Input: part model. Units: mm. Frame: model coordinates. A direction names the side the tool comes from. Round coordinates to 2 decimals unless told otherwise and drop trailing zeros. Loops run counter-clockwise (first coordinate to the right, second up) from the corner with the lowest first, then second, coordinate; pieces in that order, holes last.
(1) Cut plane C-C, the plane y = -10. Output: boundary loops of the cut face in (x, z), and give its area (3 significant figures).
(2) Cut plane D-D, the plane x = -26. Output: boundary loops of the cut face in (y, z), and give its area (3 significant figures).
(3) Draft query along X for faces 5 (the face through (11, 45, 0)), 6 (the face through (-23.122, 11.339, -30.156)), 7 (the face through (-3.905, 42.458, -0.867)). Return one class per face: released by +X, released by -X, zero draft, split by the parting line, or undercut.
(4) Access query for faces 1 (the face through (-10, 33, -3)), 2 (the face through (5.554, 36.204, -13.394)), 3 (the face through (-5.265, -13.804, -3.577)), 4 (the face through (-11, 45, 0)). Directions: +Z, -Z, +X, -X, +Y, -Y. A direction counts if a zero-diameter tool reaches every point of the face in a straight line with its end or side. Return the directions, or none.
(5) Cut plane B-B, the plane x = 0. Output: boundary loops of the cut face in (y, z).
(6) Line query: line 1 (Y direction, x = -9, z = 8); line 2 (Y direction, x = 11, z = 7); line 3 (Y direction, x = 7, z = -23). Output: solid intervals per line, ascending.
(7) First-contact query: pin 1 Ø12 at (y, z) = (-44.5, 18) entering from -X; pin 2 Ø6 at (x, z) = (7.5, -5.5) entering from +Y; pin 3 Ø2.5 at (x, z) = (11.5, 0.5) entering from +Y; pin 4 Ø23 at (x, z) = (5.5, -1) entering from +Y. Flat tips, straight axial feed; report the tip coordinate or a pass-through.
from build123d import *

# Parameters (mm, degrees)
SKETCH_1_R      = 38
EXTRUDE_1_DEPTH = 23
SKETCH_2_R      = 10
EXTRUDE_2_DEPTH = 10
SKETCH_3_R      = 14.5
EXTRUDE_3_DEPTH = 6.5
SKETCH_4_R      = 4
EXTRUDE_4_DEPTH = 6
SKETCH_5_R      = 1.5
EXTRUDE_5_DEPTH = 5.5
SKETCH_6_R      = 16.5
EXTRUDE_6_DEPTH = 28
SKETCH_7_R      = 15
EXTRUDE_7_DEPTH = 30


with BuildPart() as part:
    # Эскиз1 → Вытянуть1 (new body)
    with BuildSketch(Plane(origin=(0, 0, 0), x_dir=(1, 0, 0), z_dir=(0, 1, 0))):
        with Locations(Location((0, 0, 0), (0, 0, 270))):
            Circle(SKETCH_1_R)
    extrude(amount=EXTRUDE_1_DEPTH)

    # Эскиз2 → Вытянуть2 (add)
    with BuildSketch(Plane(origin=(0, 23, 0), x_dir=(1, 0, 0), z_dir=(0, 1, 0))):
        with Locations(Location((0, 0, 0), (0, 0, 270))):
            Circle(SKETCH_2_R)
    extrude(amount=EXTRUDE_2_DEPTH)

    # Эскиз3 → Вытянуть3 (add)
    with BuildSketch(Plane(origin=(0, 33, 0), x_dir=(1, 0, 0), z_dir=(0, 1, 0))):
        with Locations(Location((0, 0, 0), (0, 0, 90))):
            Circle(SKETCH_3_R)
    extrude(amount=EXTRUDE_3_DEPTH)

    # Эскиз4 → Вытянуть4 (add)
    with BuildSketch(Plane(origin=(0, 39.5, 0), x_dir=(-1, 0, 0), z_dir=(0, 1, 0))):
        with Locations(Location((0, 0, 0), (0, 0, 90))):
            Circle(SKETCH_4_R)
    extrude(amount=EXTRUDE_4_DEPTH)

    # Эскиз5 → Вытянуть5 (add)
    with BuildSketch(Plane(origin=(0, 39.5, 0), x_dir=(-1, 0, 0), z_dir=(0, 1, 0))):
        with Locations(Location((11, 0, 0), (0, 0, 90))):
            Circle(SKETCH_5_R)
        with Locations(Location((-11, 0, 0), (0, 0, 90))):
            Circle(SKETCH_5_R)
    extrude(amount=EXTRUDE_5_DEPTH)

    # Эскиз6 → Вытянуть6 (add)
    with BuildSketch(Plane.XZ):
        with Locations(Location((-21.372740523, 0, 0), (0, 0, 90))):
            Circle(SKETCH_6_R)
    extrude(amount=EXTRUDE_6_DEPTH)

    # Эскиз7 → Вытянуть7 (add)
    with BuildSketch(Plane.XZ.offset(28)):
        with Locations(Location((-21.372740523, 0, 0), (0, 0, 270))):
            Circle(SKETCH_7_R)
    extrude(amount=EXTRUDE_7_DEPTH)


solid = part.part
Reported:
1. outline: circle Ø33 at (-21.37, 0)
1. area: 855 mm2
2. outline: (-58, -14.27) - (-28, -14.27) - (-28, -15.84) - (0, -15.84) - (0, -27.71) - (23, -27.71) - (23, 27.71) - (0, 27.71) - (0, 15.84) - (-28, 15.84) - (-28, 14.27) - (-58, 14.27) - close
2. area: 3,020 mm2
3. face 5: zero draft
3. face 6: split by the parting line
3. face 7: undercut
4. face 1: none
4. face 2: +Y
4. face 3: -Y
4. face 4: +Z, -Z, -X, +Y
5. outline: (0, -38) - (23, -38) - (23, -10) - (33, -10) - (33, -14.5) - (39.5, -14.5) - (39.5, -4) - (45.5, -4) - (45.5, 4) - (39.5, 4) - (39.5, 14.5) - (33, 14.5) - (33, 10) - (23, 10) - (23, 38) - (0, 38) - close
6. line 1: y = -58 to 23, 33 to 39.5
6. line 2: y = 0 to 23, 33 to 39.5
6. line 3: y = 0 to 23
7. pin 1: stops at x = -30.37
7. pin 2: stops at y = 39.5
7. pin 3: stops at y = 45
7. pin 4: stops at y = 45.5
